Verification items for the finished model (mm, model axes). Face numbers are marked on the shaded views. A direction names the side the tool comes from. Give positions to 0.01 mm unless a question says otherwise; leave off trailing zeros. Loops run counter-clockwise (first coordinate to the right, second up) from the corner with the lowest first, then second, coordinate; pieces in that order, holes last. Notation, with made-up numbers: (86, -17.75) - (130, -17.75) arc R27 ccw to (130, 7.25) - close; hole circle Ø4 at (10.25, -15). An arc over 180 degrees is marked (long way). Answer in a Markdown table with one row per item.
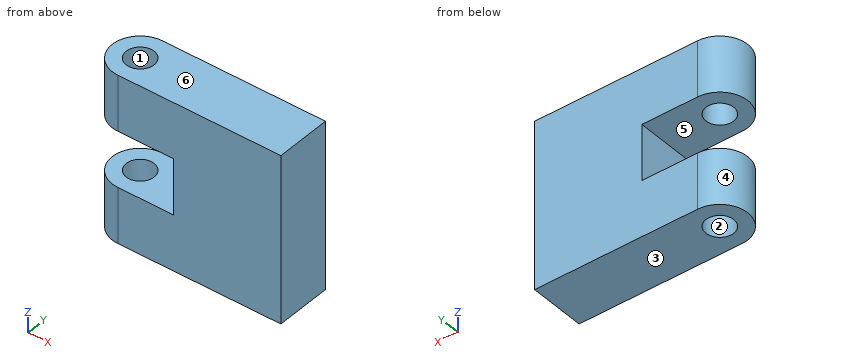
```python
from build123d import *

# Parameters (mm, degrees)
SKETCH1_R               = 10
BOSS_EXTRUDE1_DEPTH     = 60
CUT_EXTRUDE1_DEPTH      = 20
CUT_EXTRUDE1_DEPTH_BACK = 40
SKETCH2_W               = 20
SKETCH2_H               = 28.944782362
SKETCH3_R               = 5
CUT_EXTRUDE3_DEPTH      = 120
SKETCH4_W               = 60
SKETCH4_H               = 20
BOSS_EXTRUDE2_DEPTH     = 5


with BuildPart() as part:
    # Sketch1 → Boss-Extrude1 (new body)
    with BuildSketch(Plane.XY):
        Circle(SKETCH1_R)
        with BuildLine():
            Line((53.512258846, 10), (0, 10))
            ThreePointArc((0, 10), (7.071067812, 7.071067812), (10, 0))
            ThreePointArc((10, 0), (7.071067812, -7.071067812), (0, -10))
            Line((0, -10), (53.512258846, -10))
            Line((53.512258846, -10), (53.512258846, 10))
        make_face()
    extrude(amount=BOSS_EXTRUDE1_DEPTH)

    # Sketch2 → Cut-Extrude1 (cut, two sides: drawn at the far end of the back side and taken through both)
    with BuildSketch(Plane(origin=(0, 0, 0), x_dir=(0, 0, -1), z_dir=(1, 0, 0)).offset(-CUT_EXTRUDE1_DEPTH_BACK)):
        with Locations((-30, 0)):
            Rectangle(SKETCH2_W, SKETCH2_H)
    extrude(amount=CUT_EXTRUDE1_DEPTH + CUT_EXTRUDE1_DEPTH_BACK, mode=Mode.SUBTRACT)

    # Sketch3 → Cut-Extrude3 (cut)
    with BuildSketch(Plane.XY.offset(60)):
        Circle(SKETCH3_R)
    extrude(amount=-CUT_EXTRUDE3_DEPTH, mode=Mode.SUBTRACT)

    # Sketch4 → Boss-Extrude2 (add)
    with BuildSketch(Plane(origin=(53.512258846, 0, 0), x_dir=(0, 0, -1), z_dir=(1, 0, 0))):
        with Locations((-30, 0)):
            Rectangle(SKETCH4_W, SKETCH4_H)
    extrude(amount=BOSS_EXTRUDE2_DEPTH)


solid = part.part
```
Q1. Tool access check on the marked faces 5 and 6. Record the directions out of +Z, -Z, +X, -X, +Y, -Y that give a thin tool (end or side, any length) a straight path to the whole face; none if there is none.
Completed:
| item | result |
|---|---|
| face 5 | -X, +Y, -Y |
| face 6 | +Z, +X, -X, +Y, -Y |
Q2. Thickness scan on line 1 (Y direction, x = 0, z = 56); line 2 (Z direction, x = -2.5, y = 4.5); line 3 (X direction, y = -2.25, z = 33.5). Record the ranges inside material, lowest first.
Completed:
| item | result |
|---|---|
| line 1 | -10 to -5, 5 to 10 |
| line 2 | 0 to 20, 40 to 60 |
| line 3 | 20 to 58.51 |
Q3. Sectioned sample at B-B (z = 51). Record the cut outline in (x, y), and give its area (3 significant figures).
Completed:
| item | result |
|---|---|
| outline | (0, -10) - (58.51, -10) - (58.51, 10) - (0, 10) arc R10 ccw to start; hole circle Ø10 at (0, 0) |
| area | 1,250 mm^2 |
Q4. Go/stop test with a flat-tipped pin: P1, Ø6, axis at y = -1, z = 25.5, coming from the -X side. Record where the tip stops, or that it passes through.
Completed:
| item | result |
|---|---|
| P1 | x = 20 |
Q5. Sectioned sample at C-C (y = 6.75). Record the cut outline in (x, z), and give its area (3 significant figures).
Completed:
| item | result |
|---|---|
| outline | (-7.38, 0) - (58.51, 0) - (58.51, 60) - (-7.38, 60) - (-7.38, 40) - (20, 40) - (20, 20) - (-7.38, 20) - close |
| area | 3,410 mm^2 |
Q6. Draft check along X on the marked faces 1, 2, 3 and 4. Enter one of: +X half, -X half, draft (parallel to the pull), parting line (faces both ways), or undercut.
Completed:
| item | result |
|---|---|
| face 1 | undercut |
| face 2 | undercut |
| face 3 | draft |
| face 4 | -X half |
Q7. Sectioned sample at A-A (y = 0). Record the cut outline in (x, z).
Completed:
| item | result |
|---|---|
| outline | (-10, 0) - (-5, 0) - (-5, 20) - (-10, 20) - close; (-10, 40) - (-5, 40) - (-5, 60) - (-10, 60) - close; (5, 0) - (58.51, 0) - (58.51, 60) - (5, 60) - (5, 40) - (20, 40) - (20, 20) - (5, 20) - close |
Q8. Sectioned sample at D-D (z = 26). Record the cut outline in (x, y).
Completed:
| item | result |
|---|---|
| outline | (20, -10) - (58.51, -10) - (58.51, 10) - (20, 10) - close |
